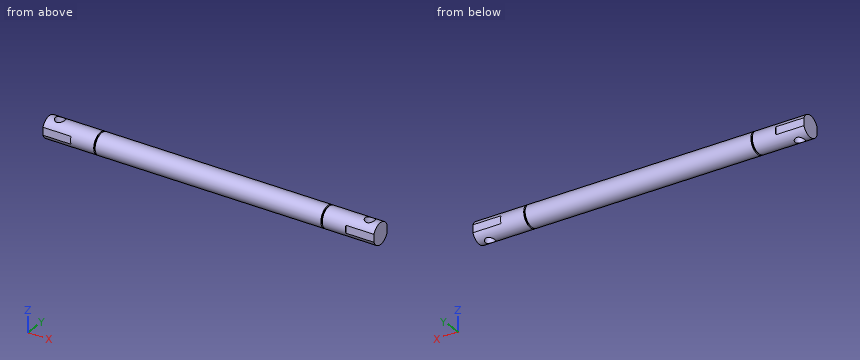
```python
from build123d import *

# Parameters (mm, degrees)
IZIM1_R                     = 7.5
Y_KSEKLIK_EKSTR_ZYON1_DEPTH = 118
IZIM2_W                     = 1
IZIM2_H                     = 2
KES_EKSTR_ZYON1_DEPTH       = 20
M8_DI_LI_DELIK1_D           = 6.8
AYNALAMA3_COPY_1_DEPTH      = 20


with BuildPart() as part:
    # Çizim1 → Yükseklik-Ekstrüzyon1 (new, symmetric)
    with BuildSketch(Plane(origin=(0, 0, 0), x_dir=(0, 0, -1), z_dir=(1, 0, 0))):
        Circle(IZIM1_R)
    extrude(amount=Y_KSEKLIK_EKSTR_ZYON1_DEPTH, both=True)

    # Çizim2 → Kes-Döndür2 (revolve, cut)
    with BuildSketch(Plane.XY, mode=Mode.PRIVATE) as kes_d_nd_r2_sk:
        with Locations((-81, 7.5)):
            Rectangle(IZIM2_W, IZIM2_H)
    kes_d_nd_r2 = revolve(kes_d_nd_r2_sk.sketch.rotate(Axis((0, 0, 0), (-1, 0, 0)), 90), axis=Axis((0, 0, 0), (-1, 0, 0)), mode=Mode.SUBTRACT)

    # Çizim3 → Kes-Ekstrüzyon1 (cut)
    with BuildSketch(Plane.ZY.offset(118)):
        Polygon((5.217035769, 7), (-5.217035769, 7), (-0.675959806, 12.212790329), align=None)
    kes_ekstr_zyon1 = extrude(amount=-KES_EKSTR_ZYON1_DEPTH, mode=Mode.SUBTRACT)

    # Aynalama2: Kes-Ekstrüzyon1 across plane
    add(kes_ekstr_zyon1.mirror(Plane.ZX), mode=Mode.SUBTRACT)

    # M8 Dişli Delik1 (through all)
    with Locations(Plane.XY.offset(12)):
        with Locations((-110.5, 0)):
            m8_di_li_delik1 = Hole(M8_DI_LI_DELIK1_D / 2)

    # Aynalama3: Kes-Döndür2, Kes-Ekstrüzyon1, M8 Dişli Delik1 across plane
    add(kes_d_nd_r2.mirror(Plane(origin=(0, 0, 0), x_dir=(0, 0, 1), z_dir=(1, 0, 0))), mode=Mode.SUBTRACT)
    add(kes_ekstr_zyon1.mirror(Plane(origin=(0, 0, 0), x_dir=(0, 0, 1), z_dir=(1, 0, 0))), mode=Mode.SUBTRACT)
    add(m8_di_li_delik1.mirror(Plane(origin=(0, 0, 0), x_dir=(0, 0, 1), z_dir=(1, 0, 0))), mode=Mode.SUBTRACT)

    # Aynalama3 copy 1 sketch → Aynalama3 copy 1 (cut)
    with BuildSketch(Plane(origin=(118, 0, 0), x_dir=(0, 0, 1), z_dir=(1, 0, 0))):
        Polygon((5.217035769, 7), (-5.217035769, 7), (-0.675959806, 12.212790329), align=None)
    extrude(amount=-AYNALAMA3_COPY_1_DEPTH, mode=Mode.SUBTRACT)


solid = part.part
```
For this review, take the finished solid that the model builds, in its own axes (mm). Round coordinates to 2 decimals unless told otherwise and drop trailing zeros. Write each loop counter-clockwise with the first axis right and the second up, starting at its lowest first coordinate (ties: lowest second). Pieces come first, ordered by that corner, then holes. Notation, with made-up numbers: (-30, 85.5) - (-15, 85.5) arc R36 ccw to (-15, 123.5) - close; hole circle Ø7 at (79, 7). An arc over 180 degrees is marked (long way). Answer as CSV lines item,"result". Start each with the question number.
(1) For line 1 (X direction, y = 0, z = 0); line 2 (X direction, y = -6.5, z = -2); line 3 (Y direction, x = -110.5, z = 1.75), list the stretches that pass through material, from the lowest coordinate up.
(2) Add section B-B, the plane x = -110.5. State the section outline as (y, z) points, plus the area to 3 significant figures.
(3) Add section C-C, the plane x = 6.5. State the section outline as (y, z) points.
(4) Add section A-A, the plane z = 0. State how many separate pieces and enclosed holes the cut face has, plus the area to 3 significant figures.
(5) For pin 1 (4 mm diameter, centred on x = 110.5, y = 0, fed in from +Z); pin 2 (3 mm diameter, centred on x = 51, z = 5.5, fed in from -Y); pin 3 (1.6 mm diameter, centred on x = 112.5, z = 1, fed in from -Y); pin 4 (0.6 mm diameter, centred on y = -7.5, z = -1, fed in from +X), all flat-tipped, find the tip position at first contact; note any pin that passes through.
From the geometry:
1,line 1,"x = -118 to -113.9, -107.1 to 107.1, 113.9 to 118"
1,line 2,"x = -118 to -81.5, -80.5 to 80.5, 81.5 to 118"
1,line 3,"y = -7 to -3.4, 3.4 to 7"
2,outline,"(-7, -2.69) arc R7.5 ccw to (-3.4, -6.69) - (-3.4, 6.69) arc R7.5 ccw to (-7, 2.69) - close; (3.4, -6.69) arc R7.5 ccw to (7, -2.69) - (7, 2.69) arc R7.5 ccw to (3.4, 6.69) - close"
2,area,"74.7 mm²"
3,outline,"circle Ø15 at (0, 0)"
4,separate pieces,"1"
4,enclosed holes,"2"
4,area,"3,420 mm²"
5,pin 1,"passes through"
5,pin 2,"stops at y = -6.34"
5,pin 3,"stops at y = -7"
5,pin 4,"stops at x = 98"
